Geometry: final body of the model. Coordinates: model frame, mm. A direction names the side the tool comes from. Round coordinates to 2 decimals unless told otherwise and drop trailing zeros. Loops run counter-clockwise (first coordinate to the right, second up) from the corner with the lowest first, then second, coordinate; pieces in that order, holes last. Notation, with made-up numbers: M 36.5,47.25 L 72.5,47.25 A7 cw 72.5,54.25 Z; hole C 38.25,34.5 d6. An arc over 180 degrees is marked long. Answer as a JSON object with one key per item and string values.
```python
from build123d import *

# Parameters (mm, degrees)
CBORE_FOR_M4_SHCS3_D           = 4.5
CBORE_FOR_M4_SHCS3_CBORE_D     = 8
CBORE_FOR_M4_SHCS3_CBORE_DEPTH = 4.2
CBORE_FOR_M4_SHCS4_D           = 4.5
CBORE_FOR_M4_SHCS4_CBORE_D     = 8
CBORE_FOR_M4_SHCS4_CBORE_DEPTH = 4


with BuildPart() as part:
    # Sketch1 → Revolve1 (revolve)
    with BuildSketch(Plane(origin=(0, 0, 0), x_dir=(0, 0, -1), z_dir=(1, 0, 0)), mode=Mode.PRIVATE) as revolve1_sk:
        Polygon((-12.75, 0), (-45.75, 0), (-45.75, 8), (-20.75, 8), (-20.75, 30), (-12.75, 30), align=None)
    revolve(revolve1_sk.sketch.rotate(Axis((0, -55, 0), (0, 1, 0)), 180), axis=Axis((0, -55, 0), (0, 1, 0)))

    # CBORE for M4 SHCS3 (through all)
    with Locations(Plane(origin=(0, 8, 0), x_dir=(1, 0, 0), z_dir=(0, 1, 0))):
        with Locations((0, 33.25), (28.795344676, 16.625), (28.795344676, -16.625), (0, -33.25), (-28.795344676, -16.625), (-28.795344676, 16.625)):
            CounterBoreHole(CBORE_FOR_M4_SHCS3_D / 2, CBORE_FOR_M4_SHCS3_CBORE_D / 2, CBORE_FOR_M4_SHCS3_CBORE_DEPTH)

    # CBORE for M4 SHCS4 (through all)
    with Locations(Plane(origin=(0, 8, 0), x_dir=(1, 0, 0), z_dir=(0, 1, 0))):
        with Locations((15.313173529, 29.513881759), (-15.313173529, -29.513881759)):
            CounterBoreHole(CBORE_FOR_M4_SHCS4_D / 2, CBORE_FOR_M4_SHCS4_CBORE_D / 2, CBORE_FOR_M4_SHCS4_CBORE_DEPTH)


solid = part.part
```
1) Set-up query: faces 1 (the face through (14.1, 1.97, -31.41)), 2 (the face through (-24.98, 5.93, -17.83)). Return all of +Z, -Z, +X, -X, +Y, -Y with unobstructed straight access to the full face (end or side cutting, diameter ignored); none if empty.
Geometry results:
{"face 1": "+Y, -Y", "face 2": "+Y"}
2) Cut plane C-C on y = 9.5. Return the cut outline in (x, z).
Geometry results:
{"outline": "C 0,0 d41.5; hole C 0,0 d25.5"}
3) First-contact query: pin 1 (4 mm diameter, centred on x = 28.5, z = 15.5, fed in from +Y); pin 2 (7 mm diameter, centred on x = -15.31, z = 29.51, fed in from -Y); pin 3 (4 mm diameter, centred on y = 20.5, z = -1, fed in from +X); pin 4 (5 mm diameter, centred on y = 12, z = -15, fed in from -X). Flat tips, straight axial feed; report the tip coordinate or a pass-through.
Geometry results:
{"pin 1": "y = 3.8", "pin 2": "y = 0", "pin 3": "x = 20.75", "pin 4": "x = -16.56"}
4) Cut plane B-B on z = 0. Return the cut outline in (x, y), and give its area (3 significant figures).
Geometry results:
{"outline": "M -45.75,0 L -12.75,0 L -12.75,30 L -20.75,30 L -20.75,8 L -45.75,8 Z; M 12.75,0 L 45.75,0 L 45.75,8 L 20.75,8 L 20.75,30 L 12.75,30 Z", "area": "880 mm2"}
5) Cut plane D-D on z = 24. Return the cut outline in (x, y).
Geometry results:
{"outline": "M -38.95,0 L 38.95,0 L 38.95,8 L -38.95,8 Z"}
6) Cut plane A-A on x = 0. Return the cut outline in (y, z), and give its area (3 significant figures).
Geometry results:
{"outline": "M 0,-45.75 L 8,-45.75 L 8,-37.25 L 3.8,-37.25 L 3.8,-35.5 L 0,-35.5 Z; M 0,-31 L 3.8,-31 L 3.8,-29.25 L 8,-29.25 L 8,-20.75 L 30,-20.75 L 30,-12.75 L 0,-12.75 Z; M 0,12.75 L 30,12.75 L 30,20.75 L 8,20.75 L 8,29.25 L 3.8,29.25 L 3.8,31 L 0,31 Z; M 0,35.5 L 3.8,35.5 L 3.8,37.25 L 8,37.25 L 8,45.75 L 0,45.75 Z", "area": "779 mm2"}
7) Pull-direction query (Z, two-part tool) for faces 3 (the face through (-6.2, 19.2, -19.8)), 4 (the face through (10, 0, 10)), 5 (the face through (-27, 3.8, -15)); classes: +Z half, -Z half, draft (parallel to the pull), parting line (faces both ways), or undercut.
Geometry results:
{"face 3": "parting line", "face 4": "draft", "face 5": "undercut"}
8) Line query: probe 1 along Z at (x, y) = (-1, 5); probe 2 along Z at (x, y) = (-3, 6); probe 3 along Y at (x, z) = (-29.5, -14). Output: solid intervals per line, ascending.
Geometry results:
{"probe 1": "-45.74 to -37.12, -29.38 to -12.71, 12.71 to 29.38, 37.12 to 45.74", "probe 2": "-45.65 to -35.9, -30.6 to -12.39, 12.39 to 30.6, 35.9 to 45.65", "probe 3": "0 to 3.8"}
